```python
from build123d import *

# Parameters (mm, degrees)
ESBO_O1_R                  = 7
RESSALTO_EXTRUS_O1_DEPTH   = 14.5
CORTE_EXTRUS_O1_DEPTH      = 18.557049866
CORTE_EXTRUS_O1_DEPTH_BACK = 18.557049866
ESBO_O2_W                  = 5
ESBO_O2_H                  = 15
CORTE_EXTRUS_O2_DEPTH      = 18.557049866
CORTE_EXTRUS_O2_DEPTH_BACK = 18.557049866
ESBO_O3_R                  = 2
CHANFRO1_SIZE              = 1
CHANFRO2_SIZE              = 1


with BuildPart() as part:
    # Esboço1 → Ressalto-extrusão1 (new, symmetric)
    with BuildSketch(Plane(origin=(0, 0, 0), x_dir=(1, 0, 0), z_dir=(0, 1, 0))):
        with Locations(Location((0, 0, 0), (0, 0, 90))):
            Circle(ESBO_O1_R)
    extrude(amount=RESSALTO_EXTRUS_O1_DEPTH, both=True)

    # Esboço2 → Corte-extrusão1 (cut, two sides: drawn at the far end of the back side and taken through both)
    with BuildSketch(Plane(origin=(0, 0, 0), x_dir=(0, 0, -1), z_dir=(1, 0, 0)).offset(-CORTE_EXTRUS_O1_DEPTH_BACK)):
        with Locations((0, 7)):
            Rectangle(ESBO_O2_W, ESBO_O2_H)
    extrude(amount=CORTE_EXTRUS_O1_DEPTH + CORTE_EXTRUS_O1_DEPTH_BACK, mode=Mode.SUBTRACT)

    # Esboço3 → Corte-extrusão2 (cut, two sides: drawn at the far end of the back side and taken through both)
    with BuildSketch(Plane.XY.offset(-CORTE_EXTRUS_O2_DEPTH_BACK)):
        with Locations(Location((0, 9.5, 0), (0, 0, 90))):
            Circle(ESBO_O3_R)
    extrude(amount=CORTE_EXTRUS_O2_DEPTH + CORTE_EXTRUS_O2_DEPTH_BACK, mode=Mode.SUBTRACT)

    # Chanfro1
    chanfro1_edges = [part.edges().sort_by_distance(p)[0] for p in [
        (0, -14.5, 7),
    ]]
    chamfer(chanfro1_edges, length=CHANFRO1_SIZE)

    # Chanfro2
    chanfro2_edges = [part.edges().sort_by_distance(p)[0] for p in [
        (0, -0.5, -2.5),
        (0, -0.5, 2.5),
        (3.968626967, 14.5, -5.766281297),
        (0, 14.5, 7),
        (0, 14.5, -2.5),
        (0, 14.5, 2.5),
    ]]
    chamfer(chanfro2_edges, length=CHANFRO2_SIZE)


solid = part.part
```
CAD build for the part. Positions are in the model's coordinates, mm. A direction names the side the tool comes from. Coordinates: 2 decimals unless noted, no trailing zeros. Order: outer loops, then holes, each group sorted by start corner. A loop starts at its lowest first (then second) coordinate and runs counter-clockwise, first axis right, second up. Notation, with made-up numbers: (44, 23.25) -> (65, 23.25) arc R17 ccw to (65, 47.25) -> close; hole circle Ø8 at (33, 41). An arc over 180 degrees is marked (long way). Use one line per item in the form item = value. Start each with the question number.
1) Band-saw the part on D-D on y = 4.75. Give the cut face in (x, z), then the cut area to 3 significant figures.
2) Band-saw the part on C-C on z = 0. Give the cut face in (x, y), then the cut area to 3 significant figures.
3) Tool access for faces 1 (the flat face through (0, -0.5, 0)), 2 (the cylindrical face through (-1.983, 9.24, -4.781)): list every direction of +Z, -Z, +X, -X, +Y, -Y with a clear straight run to the whole face (end or side of a thin tool).
4) Pull direction Z, two halves, no side cores. Call faces 3 (the conical face through (0.1, 14.3, -6.2)), 4 (the flat face through (0, 14, 3)), 5 (the flat face through (0, -14.5, 0)): +Z half, -Z half, draft (parallel to the pull), parting line (faces both ways), or undercut.
5) Drill centre lines: L1, parallel to Z at x = -4.25, y = 1.5; L2, parallel to X at y = 9.5, z = 3.85; L3, parallel to X at y = 9.5, z = 5.1. Where is each one in solid material? Low to high. Write a range as [from, to].
6) Band-saw the part on A-A on x = 0. Give the cut face in (y, z), then the cut area to 3 significant figures.
7) Band-saw the part on B-B on y = 9.5. Give the cut face in (x, z), then the cut area to 3 significant figures.
8) Drop flat-ended pins along their axis: pin 1 (2 mm diameter, centred on x = -2, y = -2.5, fed in from -Z); pin 2 (5 mm diameter, centred on x = 0, y = 9.5, fed in from -Z); pin 3 (8 mm diameter, centred on y = 3.5, z = 3, fed in from -X); pin 4 (1.5 mm diameter, centred on x = 4, y = 6.5, fed in from -Z). Give the stop position or say it passes through.
Entries:
q1.outline = (-6.54, -2.5) arc R7 ccw to (6.54, -2.5) -> close; (-6.54, 2.5) -> (6.54, 2.5) arc R7 ccw to start
q1.area = 85.5 mm2
q2.outline = (-7, -13.5) -> (-6, -14.5) -> (6, -14.5) -> (7, -13.5) -> (7, -0.5) -> (-7, -0.5) -> close
q2.area = 195 mm2
q3.face_1 = +X, -X, +Y
q3.face_2 = +Z, -Z
q4.face_3 = -Z half
q4.face_4 = undercut
q4.face_5 = draft
q5.L1 = [-5.56, -2.5], [2.5, 5.56]
q5.L2 = [-5.85, -2], [2, 5.85]
q5.L3 = [-4.79, -2], [2, 4.79]
q6.outline = (-14.5, -6) -> (-13.5, -7) -> (7.5, -7) -> (7.5, -2.5) -> (0.5, -2.5) -> (-0.5, -1.5) -> (-0.5, 1.5) -> (0.5, 2.5) -> (7.5, 2.5) -> (7.5, 7) -> (-13.5, 7) -> (-14.5, 6) -> close; (11.5, -7) -> (13.5, -7) -> (14.5, -6) -> (14.5, -3.5) -> (13.5, -2.5) -> (11.5, -2.5) -> close; (11.5, 2.5) -> (13.5, 2.5) -> (14.5, 3.5) -> (14.5, 6) -> (13.5, 7) -> (11.5, 7) -> close
q6.area = 293 mm2
q7.outline = (-6.54, -2.5) arc R7 ccw to (-2, -6.71) -> (-2, -2.5) -> close; (-6.54, 2.5) -> (-2, 2.5) -> (-2, 6.71) arc R7 ccw to start; (2, -6.71) arc R7 ccw to (6.54, -2.5) -> (2, -2.5) -> close; (2, 2.5) -> (6.54, 2.5) arc R7 ccw to (2, 6.71) -> close
q7.area = 50.2 mm2
q8.pin_1 = -6.93
q8.pin_2 = -7
q8.pin_3 = -6.79
q8.pin_4 = -6.2
